The model under review builds one solid part; all positions refer to its coordinate system, in mm. Face numbers are marked on the shaded views. A direction names the side the tool comes from. Give positions to 0.01 mm unless a question says otherwise; leave off trailing zeros. Loops run counter-clockwise (first coordinate to the right, second up) from the corner with the lowest first, then second, coordinate; pieces in that order, holes last. Notation, with made-up numbers: M -13.75,-10 L 25.25,-10 A20 ccw 25.25,-2 Z; hole C 86,-37 d2. An arc over 180 degrees is marked long. Put each result on its own line as item: value. Start each with the question number.
```python
from build123d import *

# Parameters (mm, degrees)
SKETCH3_R           = 7
BOSS_EXTRUDE1_DEPTH = 4
CUT_EXTRUDE1_DEPTH  = 2
SKETCH7_R           = 1.25
CUT_EXTRUDE2_DEPTH  = 3
CUT_EXTRUDE3_DEPTH  = 10


with BuildPart() as part:
    # Sketch1 → Revolve1 (revolve)
    with BuildSketch(Plane.XY):
        Polygon((0, 10), (3.9, 10), (5.127845609, 0), (5.25063017, -1), (6.258139995, -1), (4.784725265, 11), (0, 11), align=None)
    revolve(axis=Axis((0, 10, 0), (0, 1, 0)))

    # Sketch3 → Boss-Extrude1 (add)
    with BuildSketch(Plane(origin=(0, 11, 0), x_dir=(1, 0, 0), z_dir=(0, 1, 0))):
        Circle(SKETCH3_R)
    extrude(amount=BOSS_EXTRUDE1_DEPTH)

    # Sketch5 → Cut-Extrude1 (cut)
    with BuildSketch(Plane(origin=(0, 15, 0), x_dir=(1, 0, 0), z_dir=(0, 1, 0))):
        with BuildLine():
            Line((-4.847421995, 5.05), (4.847421995, 5.05))
            ThreePointArc((4.847421995, 5.05), (7, 0), (4.847421995, -5.05))
            Line((4.847421995, -5.05), (-4.847421995, -5.05))
            ThreePointArc((-4.847421995, -5.05), (-7, 0), (-4.847421995, 5.05))
        make_face()
    extrude(amount=-CUT_EXTRUDE1_DEPTH, mode=Mode.SUBTRACT)

    # Sketch7 → Cut-Extrude2 (cut)
    with BuildSketch(Plane(origin=(0, 13, 0), x_dir=(1, 0, 0), z_dir=(0, 1, 0))):
        Circle(SKETCH7_R)
    extrude(amount=-CUT_EXTRUDE2_DEPTH, mode=Mode.SUBTRACT)

    # Sketch8 → Cut-Extrude3 (cut)
    with BuildSketch(Plane.XY):
        with BuildLine():
            Line((-3.5, 4.392195616), (3.5, 4.392195616))
            ThreePointArc((3.5, 4.392195616), (4.55, 3.342195616), (3.5, 2.292195616))
            Line((3.5, 2.292195616), (-3.5, 2.292195616))
            ThreePointArc((-3.5, 2.292195616), (-4.55, 3.342195616), (-3.5, 4.392195616))
        make_face()
    extrude(amount=CUT_EXTRUDE3_DEPTH, mode=Mode.SUBTRACT)


solid = part.part
```
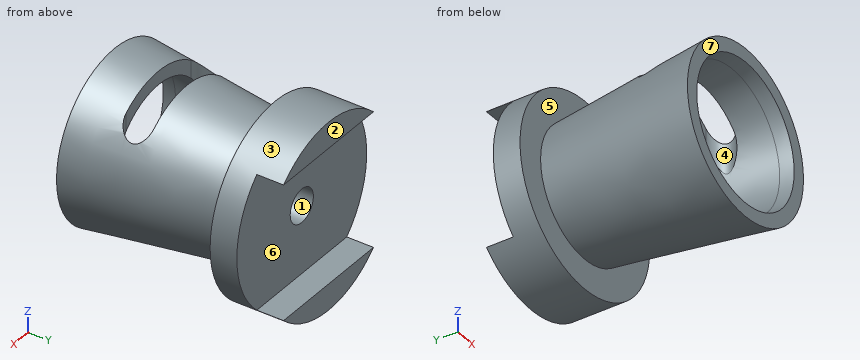
Item 1: Consider section D-D, the plane y = 3. Write out the cut boundary in (x, z), plus the area to 3 significant figures.
Item 2: Consider section A-A, the plane y = 13.75. Write out the cut boundary in (x, z).
Item 3: Tool access review of the marked faces 4, 5, 6 and 7: name each direction out of +Z, -Z, +X, -X, +Y, -Y from which nothing blocks a thin tool from reaching the whole face with its end or side.
Item 4: Consider section C-C, the plane x = -0.25. Give the number of separate pieces and of enclosed holes in the cut face, plus the area to 3 significant figures.
Item 5: Consider section B-B, the plane y = 11.5. Write out the cut boundary in (x, z), plus the area to 3 significant figures.
Item 6: Draft analysis for pull direction Z (two halves, no side actions). For the marked faces 1, 2 and 3, state which applies: +Z half, -Z half, draft (parallel to the pull), parting line (faces both ways), or undercut.
Item 7: To check wall thickness, follow L1, parallel to Z at x = 0, y = 11.65; L2, parallel to X at y = 3.75, z = 0. State the ranges of each line that lie inside material, in increasing order. Write a range as [from, to].
Item 8: Clearance check with flat-ended pins moving along their axes: pin 1 Ø1.5 at (x, z) = (0, 0) entering from +Y; pin 2 Ø6 at (x, z) = (5, 1) entering from -Y; pin 3 Ø2.5 at (x, z) = (0.5, -1.5) entering from -Y; pin 4 Ø4 at (x, y) = (0, 5.5) entering from -Z. State where each tip first meets the part, or that it passes through.
Report:
1. outline: M -4.49,1.57 L -4.49,3.62 A5.77 ccw long 4.49,3.62 L 4.49,1.57 A4.76 cw long Z
1. area: 22.4 mm²
2. outline: M -4.85,-5.05 A7 ccw 4.85,-5.05 Z; M -4.85,5.05 L 4.85,5.05 A7 ccw Z
3. face 4: +Z
3. face 5: none
3. face 6: +X, -X, +Y
3. face 7: +Z, -Z, +X, -X, -Y
4. separate pieces: 3
4. enclosed holes: 0
4. area: 58.2 mm²
5. outline: C 0,0 d14; hole C 0,0 d2.5
5. area: 149 mm²
6. face 1: undercut
6. face 2: draft
6. face 3: parting line
7. L1: [-7, -1.25], [1.25, 7]
7. L2: [-5.67, -4.67], [4.67, 5.67]
8. pin 1: through
8. pin 2: y = -1
8. pin 3: y = 10
8. pin 4: z = -5.71
